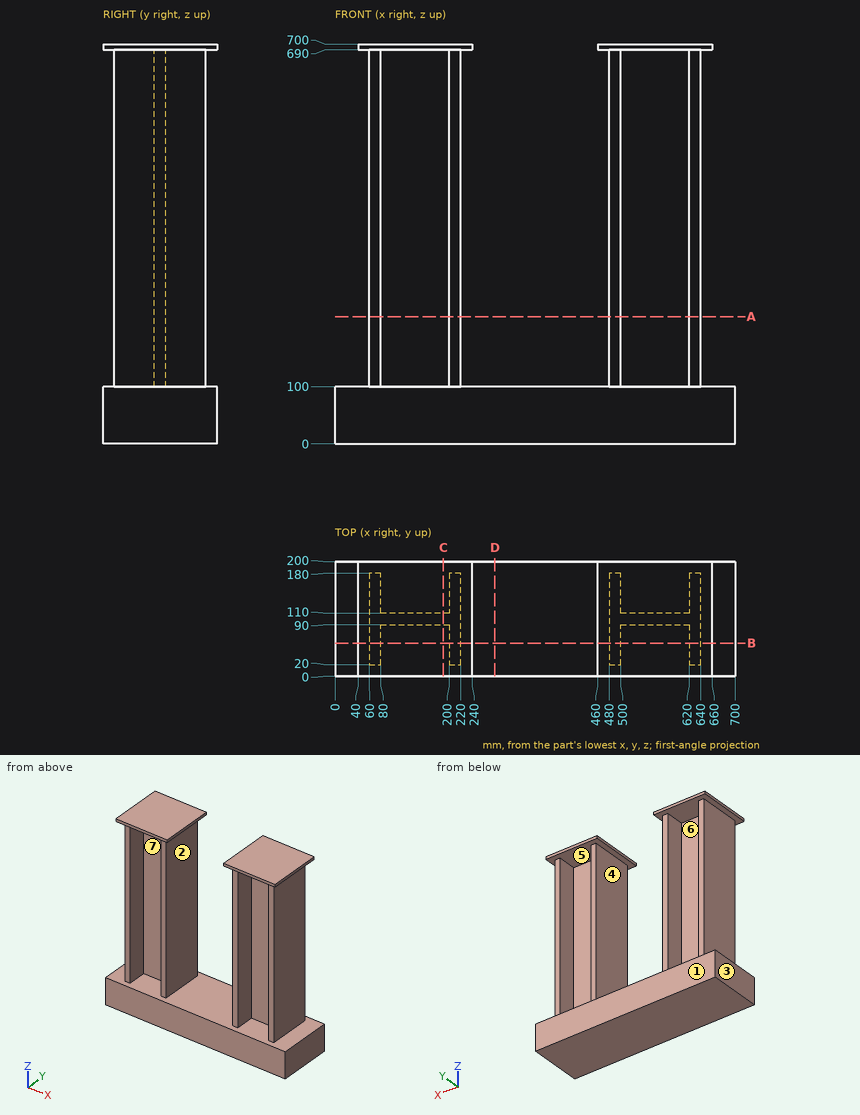
Check sheet for the drawn part. Datum: minimum x, y, z corner. Units: mm. A direction names the side the tool comes from. Give positions to 0.01 mm unless a question says otherwise; leave off trailing zeros. Order: outer loops, then holes, each group sorted by start corner. A loop starts at its lowest first (then second) coordinate and runs counter-clockwise, first axis right, second up. Notation, with made-up numbers: (5.5, -34) - (27.5, -34) arc R16 ccw to (27.5, -25) - close; hole circle Ø6 at (54, 14.5). An arc over 180 degrees is marked (long way). Answer as a JSON object with one key per item and string values.
(1) Cross-section at C-C (x = 189.5). Record the cut outline in (y, z), then the cut area to 3 significant figures.
Report:
{"outline": "(0, 0) - (200, 0) - (200, 100) - (110, 100) - (110, 690) - (200, 690) - (200, 700) - (0, 700) - (0, 690) - (90, 690) - (90, 100) - (0, 100) - close", "area": "33,800 mm^2"}
(2) Cross-section at A-A (z = 222.5). Record the cut outline in (x, y).
Report:
{"outline": "(60, 20) - (80, 20) - (80, 90) - (200, 90) - (200, 20) - (220, 20) - (220, 180) - (200, 180) - (200, 110) - (80, 110) - (80, 180) - (60, 180) - close; (480, 20) - (500, 20) - (500, 90) - (620, 90) - (620, 20) - (640, 20) - (640, 180) - (620, 180) - (620, 110) - (500, 110) - (500, 180) - (480, 180) - close"}
(3) Depth check by flat-ended pin: pin 1 Ø11 at (y, z) = (50, 696) entering from +X; pin 2 Ø10 at (x, z) = (207.5, 286.5) entering from +Y; pin 3 Ø8 at (x, y) = (429.5, 69) entering from +Z. Enter the tip coordinate at first touch or a pass-through.
Report:
{"pin 1": "x = 660", "pin 2": "y = 180", "pin 3": "z = 100"}
(4) Tool access check on the marked faces 4, 5, 6 and 7. Record the directions out of +Z, -Z, +X, -X, +Y, -Y that give a thin tool (end or side, any length) a straight path to the whole face; none if there is none.
Report:
{"face 4": "+Y, -Y", "face 5": "none", "face 6": "+Y", "face 7": "-Y"}
(5) Material ranges on line 1 (X direction, y = 134.5, z = 412.5); line 2 (Z direction, x = 539, y = 123.5); line 3 (Z direction, x = 248, y = 90.5), recorded low to high.
Report:
{"line 1": "60 to 80, 200 to 220, 480 to 500, 620 to 640", "line 2": "0 to 100, 690 to 700", "line 3": "0 to 100"}
(6) Cross-section at B-B (y = 57.5). Record the cut outline in (x, z).
Report:
{"outline": "(0, 0) - (700, 0) - (700, 100) - (640, 100) - (640, 690) - (660, 690) - (660, 700) - (460, 700) - (460, 690) - (480, 690) - (480, 100) - (220, 100) - (220, 690) - (240, 690) - (240, 700) - (40, 700) - (40, 690) - (60, 690) - (60, 100) - (0, 100) - close; hole (80, 100) - (200, 100) - (200, 690) - (80, 690) - close; hole (500, 100) - (620, 100) - (620, 690) - (500, 690) - close"}
(7) Draft check along X on the marked faces 1, 2 and 3. Enter one of: released by +X, released by -X, zero draft, split by the parting line, or undercut.
Report:
{"face 1": "zero draft", "face 2": "undercut", "face 3": "released by -X"}
(8) Cross-section at D-D (x = 279.5). Record the cut outline in (y, z).
Report:
{"outline": "(0, 0) - (200, 0) - (200, 100) - (0, 100) - close"}
